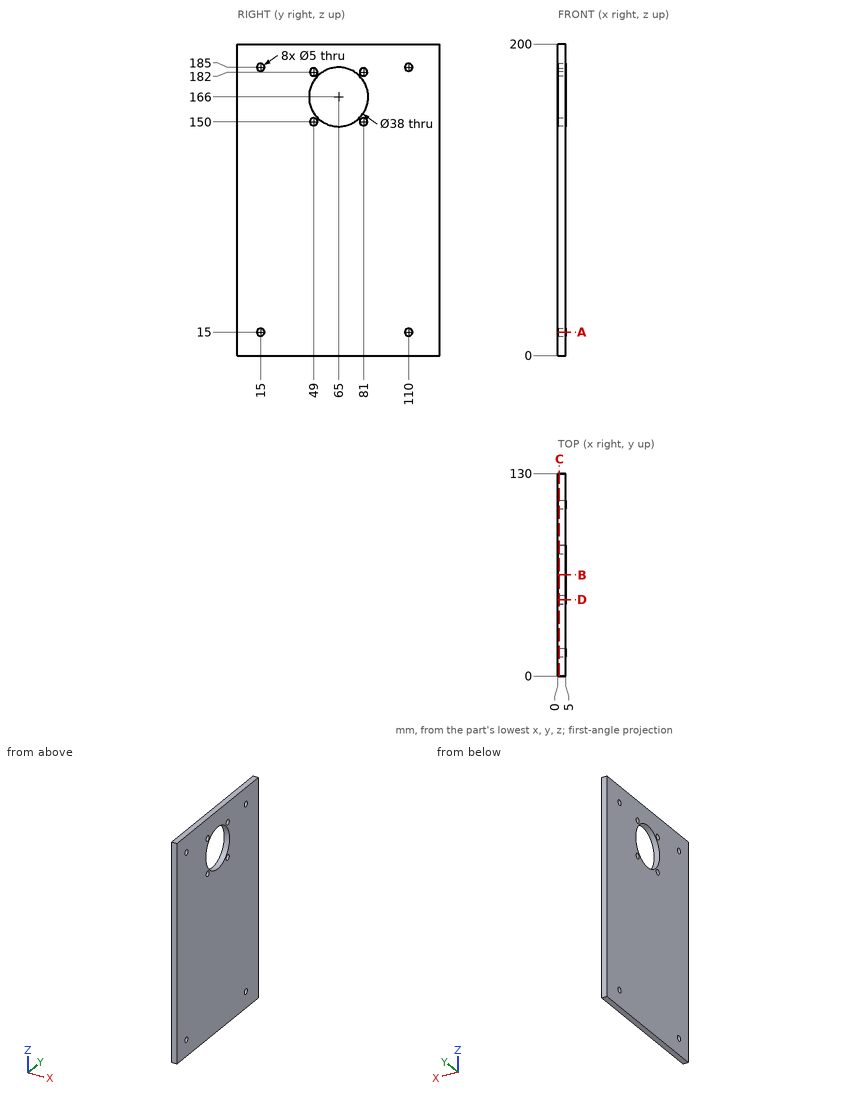
Design review of the part shown in the three views and the two pictorial views. Dimensions are in mm from the part's minimum x, y and z. Round coordinates to 2 decimals unless told otherwise and drop trailing zeros. Write each loop counter-clockwise with the first axis right and the second up, starting at its lowest first coordinate (ties: lowest second). Pieces come first, ordered by that corner, then holes. Notation, with made-up numbers: (66.5, 4) -> (96.5, 4) arc R7 cw to (96.5, 13) -> close; hole circle Ø5 at (65, 73.5). An arc over 180 degrees is marked (long way). Answer as a JSON object with one key per item and string values.
1. We need section C-C on x = 0.9. State how many separate pieces and enclosed holes the cut face has, and give its area (3 significant figures).
Results found:
{"separate pieces": "1", "enclosed holes": "9", "area": "24,700 mm^2"}
2. We need section A-A on z = 15. State the section outline as (x, y) points.
Results found:
{"outline": "(0, 0) -> (5, 0) -> (5, 12.5) -> (0, 12.5) -> close; (0, 17.5) -> (5, 17.5) -> (5, 107.5) -> (0, 107.5) -> close; (0, 112.5) -> (5, 112.5) -> (5, 130) -> (0, 130) -> close"}
3. We need section B-B on y = 65. State the section outline as (x, z) points, and give its area (3 significant figures).
Results found:
{"outline": "(0, 0) -> (5, 0) -> (5, 147) -> (0, 147) -> close; (0, 185) -> (5, 185) -> (5, 200) -> (0, 200) -> close", "area": "810 mm^2"}
4. Clearance check with a flat-ended pin moving along its axis: pin 1 (6.5 mm diameter, centred on y = 49, z = 182, fed in from -X). State where the tip first meets the part, or that it passes through.
Results found:
{"pin 1": "stops at x = 0"}
5. We need section D-D on y = 49. State the section outline as (x, z) points, and give its area (3 significant figures).
Results found:
{"outline": "(0, 0) -> (5, 0) -> (5, 147.5) -> (0, 147.5) -> close; (0, 152.5) -> (5, 152.5) -> (5, 155.75) -> (0, 155.75) -> close; (0, 176.25) -> (5, 176.25) -> (5, 179.5) -> (0, 179.5) -> close; (0, 184.5) -> (5, 184.5) -> (5, 200) -> (0, 200) -> close", "area": "848 mm^2"}
6. To check wall thickness, follow line 1 along Z through (x, y) = (1.5, 64); line 2 along Z through (x, y) = (1.5, 49); line 3 along Y through (x, z) = (2.55, 150). State the ranges of each line that lie inside material, in increasing order.
Results found:
{"line 1": "z = 0 to 147.03, 184.97 to 200", "line 2": "z = 0 to 147.5, 152.5 to 155.75, 176.25 to 179.5, 184.5 to 200", "line 3": "y = 0 to 46.5, 51.5 to 54.75, 75.25 to 78.5, 83.5 to 130"}
